Verification items for the finished model (mm, model axes). A direction names the side the tool comes from. Round coordinates to 2 decimals unless told otherwise and drop trailing zeros. Order: outer loops, then holes, each group sorted by start corner. A loop starts at its lowest first (then second) coordinate and runs counter-clockwise, first axis right, second up. Notation, with made-up numbers: M 32.5,45.25 L 67.5,45.25 A22 ccw 67.5,75.25 Z; hole C 43.5,10 d1. An arc over 180 degrees is marked long. One line per item, written item: value. Start each with the question number.
from build123d import *

# Parameters (mm, degrees)
F1_DEPTH = 22
F2_R     = 2
F3_DEPTH = 25
F5_R     = 3.5
F6_DEPTH = 8
F7_W     = 8
F7_H     = 22
F8_DEPTH = 25


with BuildPart() as f1:
    # F0 (on Front) → F1 (new body)
    with BuildSketch(Plane.XZ):
        with BuildLine():
            Line((0, 18), (-17.5, 18))
            Line((-17.5, 18), (-17.5, 13.4543560573))
            ThreePointArc((-17.5, 13.4543560573), (-14, 8), (-17.5, 2.5456439427))
            Line((-17.5, 2.5456439427), (-17.5, 0))
            Line((-17.5, 0), (0, 0))
            Line((0, 0), (0, 18))
        make_face()
    extrude(amount=F1_DEPTH)

    # F2 (on face) → F3 (cut)
    with BuildSketch(Plane(origin=(-17.5, 0, 0), x_dir=(0, -1, 0), z_dir=(-1, 0, 0))):
        with Locations((11, 8)):
            Circle(F2_R)
    extrude(amount=-F3_DEPTH, mode=Mode.SUBTRACT)

    # F5 (on face) → F6 (cut)
    with BuildSketch(Plane(origin=(-17.5, 0, 0), x_dir=(0, -1, 0), z_dir=(-1, 0, 0))):
        with Locations((11, 8)):
            Circle(F5_R)
    extrude(amount=-F6_DEPTH, mode=Mode.SUBTRACT)

    # F7 (on face) → F8 (cut)
    with BuildSketch(Plane.XY.offset(18)):
        with Locations((-4, -11)):
            Rectangle(F7_W, F7_H)
    extrude(amount=-F8_DEPTH, mode=Mode.SUBTRACT)


solid = f1.part
1. Tool access check on faces 5 (the face through (-17.5, -11, 1)), 6 (the face through (-12.4, -8.2, 5.9)). Record the directions out of +Z, -Z, +X, -X, +Y, -Y that give a thin tool (end or side, any length) a straight path to the whole face; none if there is none.
2. Section check D-D (x = -16.25). Record the cut outline in (y, z), and give its area (3 significant figures).
3. Section check B-B (z = 8). Record the cut outline in (x, y).
4. Scan lines: line 1 along Y through (x, z) = (-11.2, 8); line 2 along Z through (x, y) = (-8.95, -11); line 3 along Z through (x, y) = (-12.9, -11). Record each from-to range of solid material in increasing order.
5. Draft check along Y on faces 1 (the face through (-9.5, -13, 6)), 2 (the face through (-12, -22, 9)), 3 (the face through (-8.76, -9.526, 9.352)), 4 (the face through (-13, -11, 0)). Enter one of: released by +Y, released by -Y, zero draft, split by the parting line, or undercut.
6. Section check C-C (x = -12.75). Record the cut outline in (y, z).
7. Depth check by flat-ended pin: pin 1 (1 mm diameter, centred on y = -12.5, z = 9, fed in from +X); pin 2 (2 mm diameter, centred on y = -5.5, z = 10.5, fed in from -X); pin 3 (5 mm diameter, centred on y = -11, z = 8, fed in from -X). Enter the tip coordinate at first touch or a pass-through.
8. Section check A-A (y = -11). Record the cut outline in (x, z), and give its area (3 significant figures).
Geometry check:
1. face 5: +Z, -Z, -X, +Y, -Y
1. face 6: -X
2. outline: M -22,0 L 0,0 L 0,3.32 L -22,3.32 Z; M -22,12.68 L 0,12.68 L 0,18 L -22,18 Z
2. area: 190 mm²
3. outline: M -14,-22 L -8,-22 L -8,-13 L -9.5,-13 L -9.5,-14.5 L -14,-14.5 Z; M -14,-7.5 L -9.5,-7.5 L -9.5,-9 L -8,-9 L -8,0 L -14,0 Z
4. line 1: y = -22 to -14.5, -7.5 to 0
4. line 2: z = 0 to 6, 10 to 18
4. line 3: z = 0 to 4.5, 11.5 to 18
5. face 1: undercut
5. face 2: released by -Y
5. face 3: undercut
5. face 4: zero draft
6. outline: M -22,0 L 0,0 L 0,18 L -22,18 Z; hole C -11,8 d7
7. pin 1: stops at x = -8
7. pin 2: stops at x = -15.13
7. pin 3: stops at x = -9.5
8. outline: M -17.5,0 L -8,0 L -8,6 L -9.5,6 L -9.5,4.5 L -15.13,4.5 A6 cw -17.5,2.55 Z; M -17.5,13.45 A6 cw -15.13,11.5 L -9.5,11.5 L -9.5,10 L -8,10 L -8,18 L -17.5,18 Z
8. area: 104 mm²
